The listing builds one solid part. Answer for the finished solid, in the listing's coordinates (mm). A direction names the side the tool comes from. Coordinates: 2 decimals unless noted, no trailing zeros. Write each loop counter-clockwise with the first axis right and the second up, starting at its lowest first coordinate (ties: lowest second). Pieces come first, ordered by that corner, then holes.
from build123d import *

# Parameters (mm, degrees)
SKETCH_1_W          = 32
SKETCH_1_H          = 55
EXTRUDE_1_DEPTH     = 3
SKETCH_2_W          = 3
SKETCH_2_H          = 3
SKETCH_2_W_2        = 12
CUT_EXTRUDE_1_DEPTH = 4
SKETCH_3_W          = 3
SKETCH_3_H          = 9
CUT_EXTRUDE_2_DEPTH = 4


with BuildPart() as part:
    # 스케치1 → 보스-돌출1 (new body)
    with BuildSketch(Plane.XY):
        with Locations((16, 27.5)):
            Rectangle(SKETCH_1_W, SKETCH_1_H)
    extrude(amount=EXTRUDE_1_DEPTH)

    # 스케치2 → 컷-돌출1 (cut, through all)
    with BuildSketch(Plane.XY.offset(3)):
        with Locations((1.5, 53.5)):
            Rectangle(SKETCH_2_W, SKETCH_2_H)
        with Locations((16, 53.5)):
            Rectangle(SKETCH_2_W_2, SKETCH_2_H)
        with Locations((30.5, 53.5)):
            Rectangle(SKETCH_2_W, SKETCH_2_H)
        with Locations((1.5, 1.5)):
            Rectangle(SKETCH_2_W, SKETCH_2_H)
        with Locations((16, 1.5)):
            Rectangle(SKETCH_2_W_2, SKETCH_2_H)
        with Locations((30.5, 1.5)):
            Rectangle(SKETCH_2_W, SKETCH_2_H)
    extrude(amount=-CUT_EXTRUDE_1_DEPTH, mode=Mode.SUBTRACT)

    # 스케치3 → 컷-돌출2 (cut, through all)
    with BuildSketch(Plane.XY.offset(3)):
        with Locations((4.5, 42.5)):
            Rectangle(SKETCH_3_W, SKETCH_3_H)
        with Locations((27.5, 42.5)):
            Rectangle(SKETCH_3_W, SKETCH_3_H)
        with Locations((27.5, 12.5)):
            Rectangle(SKETCH_3_W, SKETCH_3_H)
        with Locations((4.5, 12.5)):
            Rectangle(SKETCH_3_W, SKETCH_3_H)
    extrude(amount=-CUT_EXTRUDE_2_DEPTH, mode=Mode.SUBTRACT)


solid = part.part
Q1. Determine the mould class of faces 4 (the face through (30, 52, 2)), 5 (the face through (16, 52, 2)), 6 (the face through (32, 27, 1)) for opening direction X: released by +X, released by -X, zero draft, split by the parting line, or undercut.
Answers below:
face 4: zero draft
face 5: undercut
face 6: released by +X
Q2. Which of the six approach directions +Z, -Z, +X, -X, +Y, -Y give full straight-line access (tool end or side, diameter ignored) to faces 1 (the face through (29, 53, 2)), 2 (the face through (30, 3, 2)), 3 (the face through (4, 38, 2))?
Answers below:
face 1: +Z, -Z, +X, +Y
face 2: +Z, -Z, +X, -Y
face 3: +Z, -Z
Q3. The part is cut by section C-C, the plane z = 1.6. State how many separate pieces and enclosed holes the cut face has, then the cut area to 3 significant figures.
Answers below:
separate pieces: 1
enclosed holes: 4
area: 1,540 mm2
Q4. Given pin 1 (1.5 mm diameter, centred on y = 53, z = 1.5, fed in from -X); pin 2 (0.9 mm diameter, centred on x = 17, z = 2, fed in from +Y), each flat-ended and moving along its own axis, determine where each tip first touches the part or whether it passes through.
Answers below:
pin 1: stops at x = 3
pin 2: stops at y = 52
Q5. Find the intervals of material crossed by probe 1 along X at (y, z) = (12, 2.4); probe 2 along Y at (x, z) = (27, 0.8); probe 3 along Y at (x, z) = (16, 1.9), in increasing order.
Answers below:
probe 1: x = 0 to 3, 6 to 26, 29 to 32
probe 2: y = 0 to 8, 17 to 38, 47 to 55
probe 3: y = 3 to 52
Q6. The part is cut by section A-A, the plane y = 46. Write down the section's boundary in (x, z), then the cut area to 3 significant figures.
Answers below:
outline: (0, 0) - (3, 0) - (3, 3) - (0, 3) - close; (6, 0) - (26, 0) - (26, 3) - (6, 3) - close; (29, 0) - (32, 0) - (32, 3) - (29, 3) - close
area: 78.0 mm2
Q7. The part is cut by section D-D, the plane x = 13. Write down the section's boundary in (y, z), then the cut area to 3 significant figures.
Answers below:
outline: (3, 0) - (52, 0) - (52, 3) - (3, 3) - close
area: 147 mm2
Q8. The part is cut by section B-B, the plane x = 4. Write down the section's boundary in (y, z).
Answers below:
outline: (0, 0) - (8, 0) - (8, 3) - (0, 3) - close; (17, 0) - (38, 0) - (38, 3) - (17, 3) - close; (47, 0) - (55, 0) - (55, 3) - (47, 3) - close
